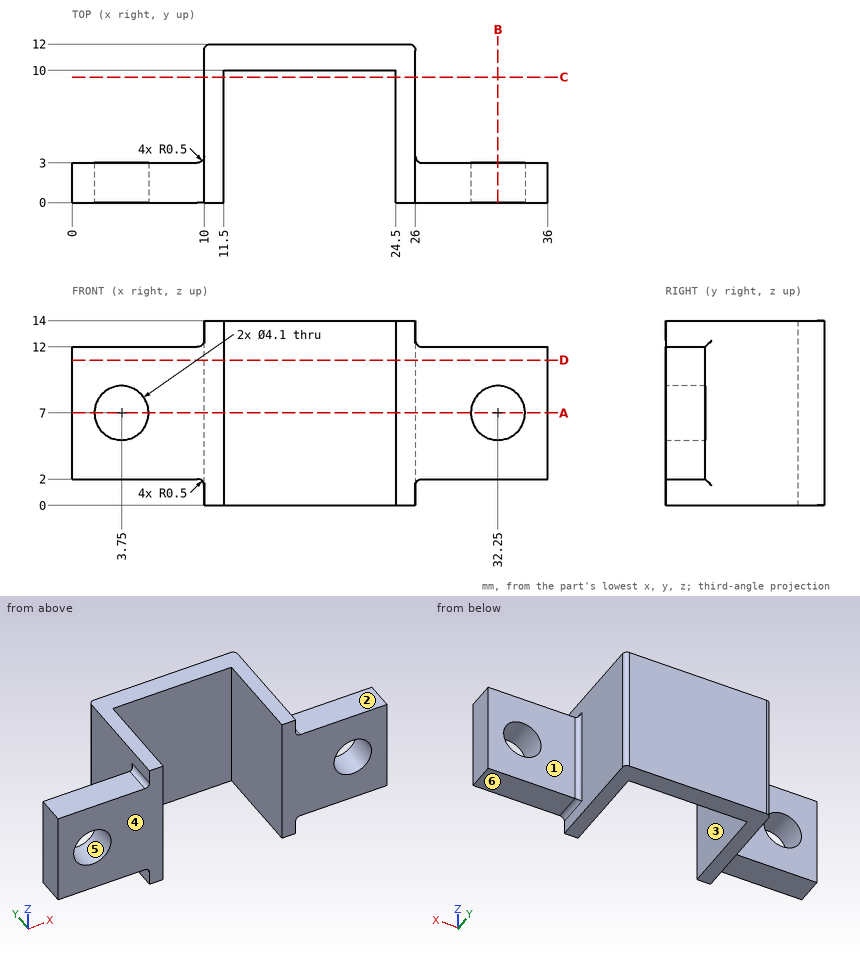
Geometry check sheet. Reference: drawing and pictorial views, mm from the part's lowest x, y, z. A direction names the side the tool comes from. Coordinates: 2 decimals unless noted, no trailing zeros. Order: outer loops, then holes, each group sorted by start corner. A loop starts at its lowest first (then second) coordinate and runs counter-clockwise, first axis right, second up.
1. Sectioned sample at C-C, the plane y = 9.5. Record the cut outline in (x, z).
Results found:
outline: (10, 0) - (11.5, 0) - (11.5, 14) - (10, 14) - close; (24.5, 0) - (26, 0) - (26, 14) - (24.5, 14) - close
2. Sectioned sample at A-A, the plane z = 7. Record the cut outline in (x, y), and give its area (3 significant figures).
Results found:
outline: (0, 0) - (1.7, 0) - (1.7, 3) - (0, 3) - close; (5.8, 0) - (11.5, 0) - (11.5, 10) - (24.5, 10) - (24.5, 0) - (30.2, 0) - (30.2, 3) - (26.5, 3) arc R0.5 cw to (26, 3.5) - (26, 11.5) arc R0.5 ccw to (25.5, 12) - (10.5, 12) arc R0.5 ccw to (10, 11.5) - (10, 3.5) arc R0.5 cw to (9.5, 3) - (5.8, 3) - close; (34.3, 0) - (36, 0) - (36, 3) - (34.3, 3) - close
area: 97.4 mm2
3. Go/stop test with flat-tipped pins: pin 1 Ø6.5 at (x, z) = (17, 7.5) entering from -Y; pin 2 Ø2.5 at (x, y) = (6, 1) entering from +Z; pin 3 Ø3 at (x, z) = (31, 5) entering from +Y; pin 4 Ø3.5 at (x, z) = (3.75, 7) entering from -Y. Record where each tip stops, or that it passes through.
Results found:
pin 1: stops at y = 10
pin 2: stops at z = 12
pin 3: stops at y = 3
pin 4: passes through
4. Release check for a two-part mould opening along Z. For the marked faces 4, 5 and 6 record: +Z half, -Z half, draft (parallel to the pull), parting line (faces both ways), or undercut.
Results found:
face 4: draft
face 5: undercut
face 6: -Z half
5. Scan lines: line 1 (X direction, y = 1.5, z = 7); line 2 (X direction, y = 7.5, z = 1.25); line 3 (X direction, y = 2.5, z = 10). Record each from-to range of solid material in increasing order.
Results found:
line 1: x = 0 to 1.7, 5.8 to 11.5, 24.5 to 30.2, 34.3 to 36
line 2: x = 10 to 11.5, 24.5 to 26
line 3: x = 0 to 11.5, 24.5 to 36
6. Sectioned sample at B-B, the plane x = 32.25. Record the cut outline in (y, z), and give its area (3 significant figures).
Results found:
outline: (0, 2) - (3, 2) - (3, 4.95) - (0, 4.95) - close; (0, 9.05) - (3, 9.05) - (3, 12) - (0, 12) - close
area: 17.7 mm2
7. Sectioned sample at D-D, the plane z = 11. Record the cut outline in (x, y), and give its area (3 significant figures).
Results found:
outline: (0, 0) - (11.5, 0) - (11.5, 10) - (24.5, 10) - (24.5, 0) - (36, 0) - (36, 3) - (26.5, 3) arc R0.5 cw to (26, 3.5) - (26, 11.5) arc R0.5 ccw to (25.5, 12) - (10.5, 12) arc R0.5 ccw to (10, 11.5) - (10, 3.5) arc R0.5 cw to (9.5, 3) - (0, 3) - close
area: 122 mm2
8. Set-up check for the marked faces 1, 2 and 3: record each of +Z, -Z, +X, -X, +Y, -Y from which the full face is reachable in a straight line by a thin tool's end or side.
Results found:
face 1: +Z, -Z, +X, +Y
face 2: +Z, +X, +Y, -Y
face 3: +Z, -Z, -Y
